```python
from build123d import *

# Parameters (mm, degrees)
SKETCH_1_W          = 44
SKETCH_1_H          = 20
EXTRUDE_1_DEPTH     = 5
SKETCH_2_W          = 7
SKETCH_2_H          = 7.6
EXTRUDE_2_DEPTH     = 30
SKETCH_3_R          = 3.3
CUT_EXTRUDE_1_DEPTH = 39.522720569
FILLET_1_R          = 6
SKETCH_4_R          = 1.6
CUT_EXTRUDE_2_DEPTH = 58.105166141


with BuildPart() as part:
    # 草图1 → 凸台-拉伸1 (new body)
    with BuildSketch(Plane(origin=(0, 0, 0), x_dir=(1, 0, 0), z_dir=(0, 1, 0))):
        Rectangle(SKETCH_1_W, SKETCH_1_H)
    extrude(amount=-EXTRUDE_1_DEPTH)

    # 草图2 → 凸台-拉伸2 (add)
    with BuildSketch(Plane.XZ.offset(5)):
        with Locations((-18.5, 0)):
            Rectangle(SKETCH_2_W, SKETCH_2_H)
        with Locations((18.5, 0)):
            Rectangle(SKETCH_2_W, SKETCH_2_H)
    extrude(amount=EXTRUDE_2_DEPTH)

    # 草图3 → 切除-拉伸1 (cut, through all)
    with BuildSketch(Plane.XZ.offset(5)):
        with Locations(Location((0, 0, 0), (0, 0, 270))):
            Circle(SKETCH_3_R)
    extrude(amount=-CUT_EXTRUDE_1_DEPTH, mode=Mode.SUBTRACT)

    # 圆角1
    fillet_1_edges = [part.edges().sort_by_distance(p)[0] for p in [
        (22, -2.5, 10),
        (-22, -2.5, 10),
        (-22, -2.5, -10),
        (22, -2.5, -10),
    ]]
    fillet(fillet_1_edges, radius=FILLET_1_R)

    # 草图4 → 切除-拉伸2 (cut, through all)
    with BuildSketch(Plane(origin=(22, 0, 0), x_dir=(0, 0, -1), z_dir=(1, 0, 0))):
        with Locations((0, -25)):
            Circle(SKETCH_4_R)
    extrude(amount=-CUT_EXTRUDE_2_DEPTH, mode=Mode.SUBTRACT)


solid = part.part
```
Verification items for the finished model (mm, model axes). A direction names the side the tool comes from. Round coordinates to 2 decimals unless told otherwise and drop trailing zeros. Order: outer loops, then holes, each group sorted by start corner. A loop starts at its lowest first (then second) coordinate and runs counter-clockwise, first axis right, second up. Notation, with made-up numbers: (-28, 8) - (-23, 8) arc R12 cw to (-23, 26) - close; hole circle Ø11 at (-6.5, -2). An arc over 180 degrees is marked (long way). Use CSV: the item, a comma, the result in double quotes. Start each with the question number.
1) Section check A-A, the plane z = 0. Record the cut outline in (x, y).
2) Access from +Z, -Z, +X, -X, +Y, -Y to the whole of each face (thin tool, end or side, straight path). Record for faces 1 (the flat face through (-22, -17, 0)), 2 (the flat face through (-19, -20, 3.8)), 3 (the flat face through (15, -20, 0)).
3) Mould release check, pull along Y, two halves, no side actions. Record for faces 4 (the cylindrical face through (20.196, -2.535, 8.289)), 5 (the cylindrical face through (-18.451, -23.414, 0.208)), 6 (the flat face through (5, 0, 0)): +Y half, -Y half, draft (parallel to the pull), parting line (faces both ways), or undercut.
4) Go/stop test with flat-tipped pins: P1, Ø2, axis at x = 20, y = -12.5, coming from the +Z side; P2, Ø3, axis at x = 9.5, z = -3.5, coming from the -Y side; P3, Ø3.5, axis at x = 20, y = -18.5, coming from the -Z side. Record where each tip stops, or that it passes through.
5) Section check B-B, the plane y = -17. Record the cut outline in (x, z), plus the area to 3 significant figures.
6) Section check D-D, the plane z = 6.75. Record the cut outline in (x, y), plus the area to 3 significant figures.
7) Thickness scan on L1, parallel to X at y = -13, z = 1.25; L2, parallel to Y at x = 10.5, z = -9; L3, parallel to Z at x = -15.5, y = -18.5. Record the ranges inside material, lowest first.
8) Section check C-C, the plane x = 0. Record the cut outline in (y, z), plus the area to 3 significant figures.
Answers:
1,outline,"(-22, -35) - (-15, -35) - (-15, -26.6) - (-22, -26.6) - close; (-22, -23.4) - (-15, -23.4) - (-15, -5) - (-3.3, -5) - (-3.3, 0) - (-22, 0) - close; (3.3, -5) - (15, -5) - (15, -23.4) - (22, -23.4) - (22, 0) - (3.3, 0) - close; (15, -35) - (22, -35) - (22, -26.6) - (15, -26.6) - close"
2,face 1,"+Z, -Z, -X, +Y, -Y"
2,face 2,"+Z, +X, -X, -Y"
2,face 3,"+Z, -Z, -Y"
3,face 4,"draft"
3,face 5,"undercut"
3,face 6,"+Y half"
4,P1,"stops at z = 3.8"
4,P2,"stops at y = -5"
4,P3,"stops at z = -3.8"
5,outline,"(-22, -3.8) - (-15, -3.8) - (-15, 3.8) - (-22, 3.8) - close; (15, -3.8) - (22, -3.8) - (22, 3.8) - (15, 3.8) - close"
5,area,"106 mm²"
6,outline,"(-21.33, -5) - (21.33, -5) - (21.33, 0) - (-21.33, 0) - close"
6,area,"213 mm²"
7,L1,"x = -22 to -15, 15 to 22"
7,L2,"y = -5 to 0"
7,L3,"z = -3.8 to 3.8"
8,outline,"(-5, -10) - (0, -10) - (0, -3.3) - (-5, -3.3) - close; (-5, 3.3) - (0, 3.3) - (0, 10) - (-5, 10) - close"
8,area,"67.0 mm²"
